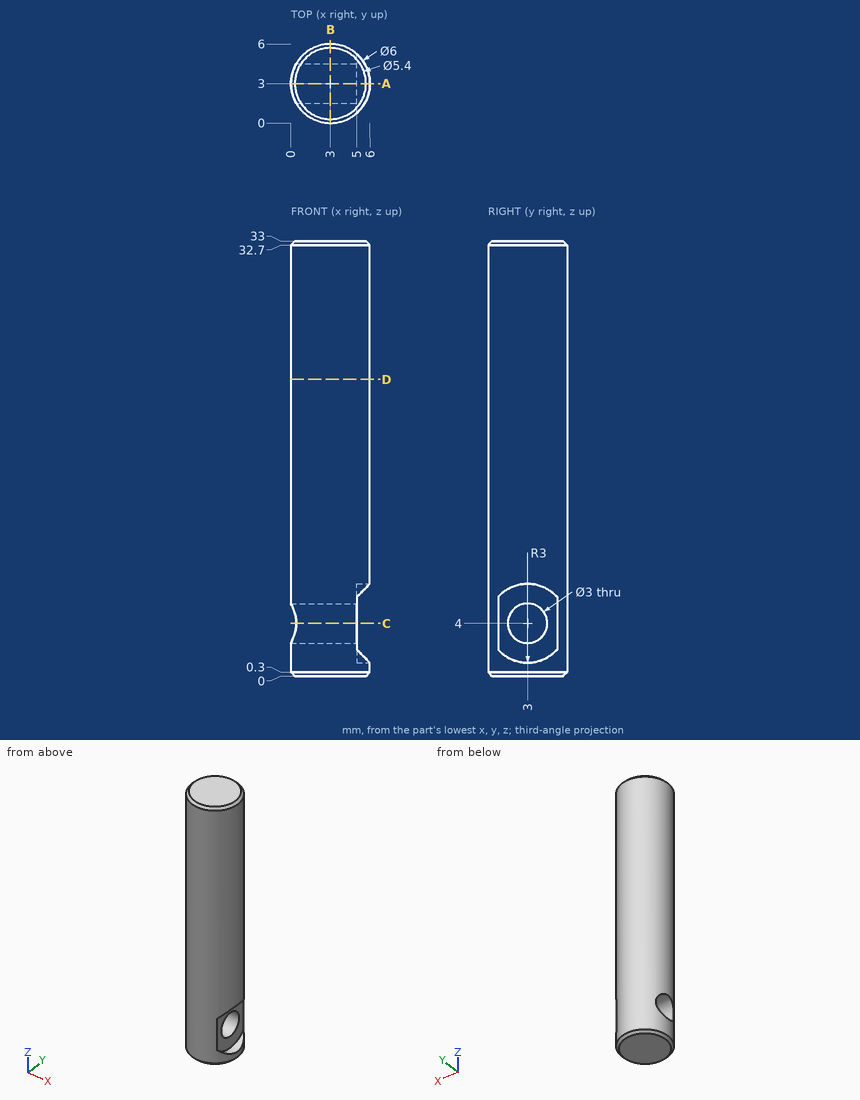
The figure shows three views and two pictorial views of one solid part (mm, origin at its lowest corner). Answer the questions. Coordinates: 2 decimals unless noted, no trailing zeros. Write each loop counter-clockwise with the first axis right and the second up, starting at its lowest first coordinate (ties: lowest second). Pieces come first, ordered by that corner, then holes.
1. The part is cut by section A-A, the plane y = 3. Write down the section's boundary in (x, z), and give its area (3 significant figures).
Results list:
outline: (0, 0.3) - (0.3, 0) - (5.7, 0) - (6, 0.3) - (6, 1) - (5, 1) - (5, 2.5) - (0, 2.5) - close; (0, 5.5) - (5, 5.5) - (5, 7) - (6, 7) - (6, 32.7) - (5.7, 33) - (0.3, 33) - (0, 32.7) - close
area: 177 mm2
2. Consider line 1 along X through (y, z) = (5, 7); line 2 along Y through (x, z) = (3.3, 4); line 3 along Z through (x, y) = (3.5, 2.25). Determine where each line is inside the solid, lowest interval first.
Results list:
line 1: x = 0.76 to 5.24
line 2: y = 0.02 to 1.5, 4.5 to 5.98
line 3: z = 0 to 2.7, 5.3 to 33
3. Flat-ended cylindrical pins translate along their axes: pin 1 (1 mm diameter, centred on y = 4, z = 18, fed in from -X); pin 2 (1.5 mm diameter, centred on x = 4.5, z = 7.5, fed in from -Y); pin 3 (3 mm diameter, centred on x = 1, z = 16.5, fed in from +Y). Find the tip coordinate at first contact, or state that the pin passes through.
Results list:
pin 1: stops at x = 0.04
pin 2: stops at y = 0.1
pin 3: stops at y = 5.96
4. The part is cut by section D-D, the plane z = 22.5. Write down the section's boundary in (x, y).
Results list:
outline: circle Ø6 at (3, 3)
5. The part is cut by section B-B, the plane x = 3. Write down the section's boundary in (y, z).
Results list:
outline: (0, 0.3) - (0.3, 0) - (5.7, 0) - (6, 0.3) - (6, 32.7) - (5.7, 33) - (0.3, 33) - (0, 32.7) - close; hole circle Ø3 at (3, 4)
6. The part is cut by section C-C, the plane z = 4. Write down the section's boundary in (x, y).
Results list:
outline: (0.4, 1.5) arc R3 ccw to (5, 0.76) - (5, 1.5) - close; (0.4, 4.5) - (5, 4.5) - (5, 5.24) arc R3 ccw to start
